from build123d import *

# Parameters (mm, degrees)
SKETCH_1_W          = 80
SKETCH_1_H          = 81
EXTRUDE_1_DEPTH     = 5
SKETCH_2_W          = 12.25
SKETCH_2_H          = 5
SKETCH_2_W_2        = 27
SKETCH_2_H_2        = 49
CUT_EXTRUDE_1_DEPTH = 10
SKETCH_5_W          = 10
SKETCH_5_H          = 5
SKETCH_5_W_2        = 5
SKETCH_5_H_2        = 10
EXTRUDE_2_DEPTH     = 5
FILLET_1_R          = 1
SKETCH_6_R          = 1.25
CUT_EXTRUDE_4_DEPTH = 10


with BuildPart() as part:
    # 스케치1 → 보스-돌출1 (new body)
    with BuildSketch(Plane.XY):
        with Locations((-45, 45.5)):
            Rectangle(SKETCH_1_W, SKETCH_1_H)
    extrude(amount=-EXTRUDE_1_DEPTH)

    # 스케치2 → 컷-돌출1 (cut)
    with BuildSketch(Plane.XY):
        with Locations((-11.125, 39.5)):
            Rectangle(SKETCH_2_W, SKETCH_2_H)
        with Locations((-45, 61.5)):
            Rectangle(SKETCH_2_W_2, SKETCH_2_H_2)
        with Locations((-78.875, 39.5)):
            Rectangle(SKETCH_2_W, SKETCH_2_H)
    extrude(amount=-CUT_EXTRUDE_1_DEPTH, mode=Mode.SUBTRACT)

    # 스케치5 → 보스-돌출2 (add)
    with BuildSketch(Plane.XY):
        with Locations((-30, 2.5)):
            Rectangle(SKETCH_5_W, SKETCH_5_H)
        with Locations((-60, 2.5)):
            Rectangle(SKETCH_5_W, SKETCH_5_H)
        with Locations((-2.5, 56)):
            Rectangle(SKETCH_5_W_2, SKETCH_5_H_2)
        with Locations((-87.5, 56)):
            Rectangle(SKETCH_5_W_2, SKETCH_5_H_2)
        with Locations((-68.5, 88.5)):
            Rectangle(SKETCH_5_W_2, SKETCH_5_H)
        with Locations((-21.5, 88.5)):
            Rectangle(SKETCH_5_W_2, SKETCH_5_H)
    extrude(amount=-EXTRUDE_2_DEPTH)

    # 필렛1
    fillet_1_edges = [part.edges().sort_by_distance(p)[0] for p in [
        (-19, 91, -2.5),
        (-66, 91, -2.5),
        (-71, 91, -2.5),
        (-24, 91, -2.5),
        (-65, 0, -2.5),
        (-35, 0, -2.5),
        (-55, 0, -2.5),
        (-25, 0, -2.5),
        (-5, 37, -2.5),
        (-5, 42, -2.5),
        (0, 61, -2.5),
        (0, 51, -2.5),
        (-85, 37, -2.5),
        (-85, 42, -2.5),
        (-90, 51, -2.5),
        (-90, 61, -2.5),
    ]]
    fillet(fillet_1_edges, radius=FILLET_1_R)

    # 스케치6 → 컷-돌출4 (cut)
    with BuildSketch(Plane.XY):
        with Locations((-32.75, 37)):
            Circle(SKETCH_6_R)
        with Locations((-57.25, 37)):
            Circle(SKETCH_6_R)
        with Locations((-74, 42)):
            Circle(SKETCH_6_R)
        with Locations((-74, 37)):
            Circle(SKETCH_6_R)
        with Locations((-16, 42)):
            Circle(SKETCH_6_R)
        with Locations((-16, 37)):
            Circle(SKETCH_6_R)
        with Locations((-5, 49.75)):
            Circle(SKETCH_6_R)
        with Locations((-5, 62.25)):
            Circle(SKETCH_6_R)
        with Locations((-85, 62.25)):
            Circle(SKETCH_6_R)
        with Locations((-85, 49.75)):
            Circle(SKETCH_6_R)
        with Locations((-66.25, 5)):
            Circle(SKETCH_6_R)
        with Locations((-53.75, 5)):
            Circle(SKETCH_6_R)
        with Locations((-36.25, 5)):
            Circle(SKETCH_6_R)
        with Locations((-23.75, 5)):
            Circle(SKETCH_6_R)
        with Locations((-72.25, 86)):
            Circle(SKETCH_6_R)
        with Locations((-64.75, 86)):
            Circle(SKETCH_6_R)
        with Locations((-25.25, 86)):
            Circle(SKETCH_6_R)
        with Locations((-17.75, 86)):
            Circle(SKETCH_6_R)
    extrude(amount=-CUT_EXTRUDE_4_DEPTH, mode=Mode.SUBTRACT)


solid = part.part
For this review, take the finished solid that the model builds, in its own axes (mm). A direction names the side the tool comes from. Coordinates: 2 decimals unless noted, no trailing zeros. Order: outer loops, then holes, each group sorted by start corner. A loop starts at its lowest first (then second) coordinate and runs counter-clockwise, first axis right, second up. Notation, with made-up numbers: (19, 16) - (77, 16) arc R18 cw to (77, 51) - close; hole circle Ø7 at (23.5, -11). An arc over 180 degrees is marked (long way). Answer as CSV lines item,"result". Start each with the question number.
1) Add section C-C (y = 12). State the section outline as (x, z) points.
2) Draft analysis for pull direction X (two halves, no side actions). For faces 4 (the flat face through (-5, 46, -2)), 5 (the cylindrical face through (-66.22, 6.25, -2.46)), 6 (the flat face through (-3, 61, -2)), state which applies: +X half, -X half, draft (parallel to the pull), parting line (faces both ways), or undercut.
3) Add section B-B (x = -82). State the section outline as (y, z) points, then the cut area to 3 significant figures.
4) Insertion check: P1, Ø2, axis at y = 88.5, z = -2, coming from the -X side; P2, Ø2.5, axis at x = -47, z = -2.5, coming from the -Y side; P3, Ø1, axis at x = -65, z = -2, coming from the -Y side; P4, Ø12, axis at x = -40.5, y = 62.5, coming from the -Z side. Each pin has a flat end and moves straight along its axis. Give the tip position at first contact, or say it passes through.
5) To check wall thickness, follow line 1 along X through (y, z) = (4.5, -1.15); line 2 along X through (y, z) = (84, -2.85); line 3 along Y through (x, z) = (-12, -1.8). State the ranges of each line that lie inside material, in increasing order. Write a range as [from, to].
6) Machinability: for faces 1 (the flat face through (-29, 86, -2)), 2 (the flat face through (-87, 51, -2)), 3 (the flat face through (-80, 42, -2)), which of the approach directions +Z, -Z, +X, -X, +Y, -Y give a long, thin tool a straight path to every point of the face, cutting with its end or side? Answer none if there is none.
7) Add section A-A (y = 49.75). State the section outline as (x, z) points, then the cut area to 4 significant figures.
Result:
1,outline,"(-85, -5) - (-5, -5) - (-5, 0) - (-85, 0) - close"
2,face 4,"+X half"
2,face 5,"undercut"
2,face 6,"draft"
3,outline,"(5, -5) - (37, -5) - (37, 0) - (5, 0) - close; (42, -5) - (86, -5) - (86, 0) - (42, 0) - close"
3,area,"380 mm^2"
4,P1,"x = -71"
4,P2,"y = 5"
4,P3,"y = 0.13"
4,P4,"through"
5,line 1,"[-65, -55], [-35, -25]"
5,line 2,"[-85, -58.5], [-31.5, -5]"
5,line 3,"[5, 37], [42, 86]"
6,face 1,"+Z, -Z, +Y"
6,face 2,"+Z, -Z, -X, -Y"
6,face 3,"+Z, -Z, -X"
7,outline,"(-83.75, -5) - (-58.5, -5) - (-58.5, 0) - (-83.75, 0) - close; (-31.5, -5) - (-6.25, -5) - (-6.25, 0) - (-31.5, 0) - close"
7,area,"252.5 mm^2"
